Model file for the job. Use its own axes, mm. Face numbers are marked on the shaded views. A direction names the side the tool comes from. Coordinates: 2 decimals unless noted, no trailing zeros. Order: outer loops, then holes, each group sorted by start corner. A loop starts at its lowest first (then second) coordinate and runs counter-clockwise, first axis right, second up. Notation, with made-up numbers: (62, 17) -> (112, 17) arc R13 ccw to (112, 35) -> close; hole circle Ø6 at (57, 64.5). An arc over 180 degrees is marked (long way). Return JSON: item names as keys, results as strings. Group by question number.
1) Pull direction Y, two halves, no side cores. Call the marked faces 3 and 4: +Y half, -Y half, draft (parallel to the pull), parting line (faces both ways), or undercut.
2) Cut at D-D (x = -42). Write the cut outline in (y, z) (3 decimals).
3) Flat gauge pins, fed straight in: pin 1 (4 mm diameter, centred on x = -12, y = -15.5, fed in from +Z); pin 2 (3.5 mm diameter, centred on x = -47, z = 4.5, fed in from +Y); pin 3 (1 mm diameter, centred on x = -20, z = 5, fed in from -Y) (3 decimals); pin 4 (4 mm diameter, centred on x = -46.5, y = -5.5, fed in from +Z) (3 decimals). Where does each tip first touch, or does it go through?
4) Probe line 1 (Y direction, x = -3, z = 6) (3 decimals); line 2 (Z direction, x = 7, y = -3.5) (3 decimals). List the from-to ranges inside material, lowest first.
5) Which spindle directions (+Z, -Z, +X, -X, +Y, -Y) get a long thin tool onto all of the face, cutting with end or side? Do the marked faces 1 and 2. Say none if no direction does.
6) Cut at C-C (y = -18.5). Write the cut outline in (x, z).
7) Cut at B-B (x = -62). Write the cut outline in (y, z) (3 decimals).
8) Cut at A-A (y = -27.94). Write the cut outline in (x, z) (3 decimals), and give its area (3 significant figures).
from build123d import *

# Parameters (mm, degrees)
F0_R     = 1.8161
F1_DEPTH = 3.175
F2_W     = 133.35
F2_H     = 15.24
F3_DEPTH = 3.175
F4_R     = 6.6675
F5_DEPTH = 0.8128


with BuildPart() as f1:
    # F0 (on Top) → F1 (new body)
    with BuildSketch(Plane.XY):
        Polygon((51.882015, -8.216515), (51.882015, 0), (-81.467985, 0), (-81.467985, -8.216515), (-81.467985, -24.110759), (-81.467985, -31.75), (51.882015, -31.75), (51.882015, -24.110759), align=None)
        with Locations((-77.657985, -27.94)):
            Circle(F0_R, mode=Mode.SUBTRACT)
        with Locations((48.072015, -27.94)):
            Circle(F0_R, mode=Mode.SUBTRACT)
        with Locations((-77.657985, -3.81)):
            Circle(F0_R, mode=Mode.SUBTRACT)
        with Locations((48.072015, -3.81)):
            Circle(F0_R, mode=Mode.SUBTRACT)
    extrude(amount=F1_DEPTH)

    # F2 (on face) → F3 (join)
    with BuildSketch(Plane.XY.offset(3.175)):
        with Locations((-14.792985, -15.875)):
            Rectangle(F2_W, F2_H)
    extrude(amount=F3_DEPTH)

    # F4 (on face) → F5 (cut)
    with BuildSketch(Plane.XY.offset(6.35)):
        with Locations((-59.242985, -15.875)):
            Circle(F4_R)
        with Locations((-14.792985, -15.875)):
            Circle(F4_R)
        with Locations((29.657015, -15.875)):
            Circle(F4_R)
    extrude(amount=-F5_DEPTH, mode=Mode.SUBTRACT)


solid = f1.part
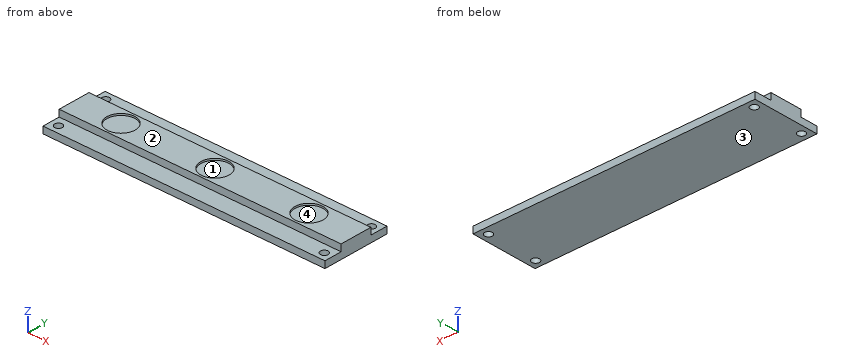
Answers below:
{
 "1": {"face 3": "draft", "face 4": "undercut"},
 "2": {"outline": "(-31.75, 0) -> (0, 0) -> (0, 3.175) -> (-8.255, 3.175) -> (-8.255, 6.35) -> (-23.495, 6.35) -> (-23.495, 3.175) -> (-31.75, 3.175) -> close"},
 "3": {"pin 1": "stops at z = 5.54", "pin 2": "stops at y = 0", "pin 3": "stops at y = -23.495", "pin 4": "stops at z = 3.175"},
 "4": {"line 1": "y = -23.495 to -8.255", "line 2": "z = 0 to 3.175"},
 "5": {"face 1": "+Z", "face 2": "+Z, +X, -X, +Y, -Y"},
 "6": {"outline": "(-81.47, 0) -> (51.88, 0) -> (51.88, 6.35) -> (35.79, 6.35) -> (35.79, 5.54) -> (23.53, 5.54) -> (23.53, 6.35) -> (-8.66, 6.35) -> (-8.66, 5.54) -> (-20.92, 5.54) -> (-20.92, 6.35) -> (-53.11, 6.35) -> (-53.11, 5.54) -> (-65.37, 5.54) -> (-65.37, 6.35) -> (-81.47, 6.35) -> close"},
 "7": {"outline": "(-31.75, 0) -> (0, 0) -> (0, 3.175) -> (-8.255, 3.175) -> (-8.255, 6.35) -> (-9.804, 6.35) -> (-9.804, 5.537) -> (-21.946, 5.537) -> (-21.946, 6.35) -> (-23.495, 6.35) -> (-23.495, 3.175) -> (-31.75, 3.175) -> close"},
 "8": {"outline": "(-81.468, 0) -> (-79.474, 0) -> (-79.474, 3.175) -> (-81.468, 3.175) -> close; (-75.842, 0) -> (46.256, 0) -> (46.256, 3.175) -> (-75.842, 3.175) -> close; (49.888, 0) -> (51.882, 0) -> (51.882, 3.175) -> (49.888, 3.175) -> close", "area": "400 mm^2"}
}
